Read the model definition and answer for the solid it produces. Units are mm, in the model's axes. Face numbers are marked on the shaded views. A direction names the side the tool comes from. Coordinates: 2 decimals unless noted, no trailing zeros. Order: outer loops, then holes, each group sorted by start corner. A loop starts at its lowest first (then second) coordinate and runs counter-clockwise, first axis right, second up. Notation, with made-up numbers: (-31, 42.25) - (-15, 42.25) arc R26 ccw to (-15, 63.25) - close; hole circle Ø3 at (-38, -29.75). An arc over 180 degrees is marked (long way). Use one line per item in the form item = value.
```python
from build123d import *

# Parameters (mm, degrees)
F0_W     = 155.6016728282
F0_H     = 72.8251989931
F1_DEPTH = 58.42
F2_W     = 155.6016728282
F2_H     = 9.92824696
F3_DEPTH = 25.4
F4_T     = 7.62
F5_R     = 5.08
F8_DEPTH = 25.4


# Not quite as in the source:
# - two fillets or chamfers of one size are made in one step
# - a shell that OpenCascade refuses in one call is made with other operations: the cavity is built on its own and cut out


with BuildPart() as f1:
    # F0 (on Front) → F1 (new body)
    with BuildSketch(Plane.XZ):
        with Locations((-1.8093250692, -6.1064558104)):
            Rectangle(F0_W, F0_H)
    extrude(amount=F1_DEPTH)

    # F2 (on face) → F3 (join)
    with BuildSketch(Plane.XY.offset(30.3061436862)):
        with Locations((-1.8093250692, -29.200729914)):
            Rectangle(F2_W, F2_H)
    extrude(amount=F3_DEPTH)

    # F4: shell of thickness 7.62, made by hand


with BuildPart() as f4_core1:
    # F4_t2: copy of F1
    add(f1.part)

    # the walls: a layer under each face that stays
    f4_faces = [f4_core1.faces().sort_by_distance(p)[0] for p in [
        (-1.8093250692, -12.118303217, 30.3061436862),
        (-1.8093250692, 0, -6.1064558104),
        (-79.6101614833, -29.21, 6.5935441896),
        (75.9915113449, -29.21, 6.5935441896),
        (-1.8093250692, -29.21, -42.5190553069),
        (-1.8093250692, -46.292426697, 30.3061436862),
        (-1.8093250692, -58.42, -6.1064558104),
        (-1.8093250692, -29.200729914, 55.7061436862),
    ]]
    thicken(f4_faces, amount=-F4_T, mode=Mode.SUBTRACT)


with BuildPart() as f1_1:
    add(f1.part)

    # what is left inside the walls is the cavity
    f4_cavity = [f4_core1.part.solids().sort_by_distance(p)[0] for p in [
        (-1.809325, -50.7238, -15.703989),
    ]]
    add(f4_cavity, mode=Mode.SUBTRACT)

    # F5
    f5_edges = [f1_1.edges().sort_by_distance(p)[0] for p in [
        (75.991511, -29.20073, 55.706144),
        (-79.610161, -29.20073, 55.706144),
    ]]
    fillet(f5_edges, radius=F5_R)

    # F7 (on face) → F8 (join)
    with BuildSketch(Plane(origin=(0, 0, 0), x_dir=(-1, 0, 0), z_dir=(0, 1, 0))):
        with BuildLine():
            Line((-33.5065312684, 8.8093429804), (-38.0396991968, 16.5818184614))
            ThreePointArc((-38.0396991968, 16.5818184614), (-46.9537485501, -29.5424136332), (0, -31.0426000506))
            ThreePointArc((0, -31.0426000506), (-11.7838373022, -4.7836219306), (-38.2480099797, -16.0991121083))
            ThreePointArc((-38.2480099797, -16.0991121083), (-40.6774615304, -20.5324220373), (-41.8258410886, -25.4556015134))
            ThreePointArc((-41.8258410886, -25.4556015134), (-44.7298971339, -6.6081053321), (-33.5065312684, 8.8093429804))
        make_face()
        with BuildLine():
            ThreePointArc((-31.2344189733, -35.0670516491), (-34.0695631474, -33.473512911), (-36.6739996827, -31.5256118532))
            ThreePointArc((-36.6739996827, -31.5256118532), (-36.1813498713, -25.629843598), (-33.3930179477, -20.4117987305))
            ThreePointArc((-33.3930179477, -20.4117987305), (-24.8135406655, -12.1786870208), (-12.9460245371, -12.9227433354))
            ThreePointArc((-12.9460245371, -12.9227433354), (-6.8355734632, -17.7428655691), (-5.7939905673, -25.4556015134))
            ThreePointArc((-5.7939905673, -25.4556015134), (-16.5679645446, -35.4128057466), (-31.2344189733, -35.0670516491))
        make_face(mode=Mode.SUBTRACT)
    extrude(amount=F8_DEPTH)


solid = f1_1.part
```
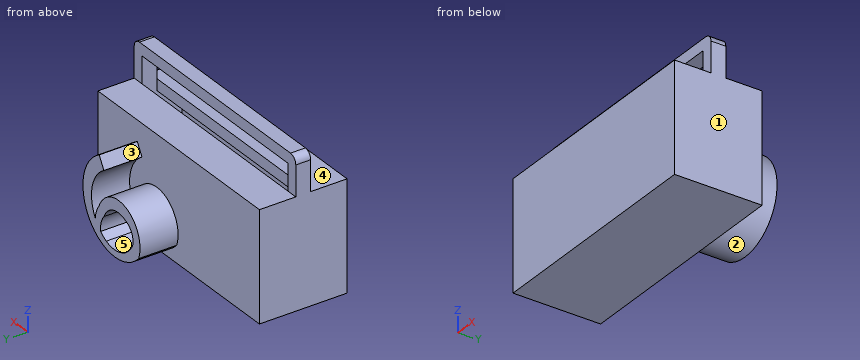
(1) Straight lines are drawn through the part: L1, parallel to Z at x = -71, y = -49.5; L2, parallel to X at y = -32.5, z = 17; L3, parallel to Y at x = 40, z = -13.5. For each, find the intervals that lie inside material, in ascending order.
Answer list:
L1 = -42.52 to -34.9, 22.69 to 30.31
L2 = -79.61 to -71.99, 68.37 to 75.99
L3 = -58.42 to -50.8, -7.62 to 0
(2) Section B-B, the plane x = -31.5 is taken. Write down the section's boundary in (y, z), then the cut area to 3 significant figures.
Answer list:
outline = (-58.42, -42.52) - (0, -42.52) - (0, 30.31) - (-24.24, 30.31) - (-24.24, 22.69) - (-7.62, 22.69) - (-7.62, -34.9) - (-50.8, -34.9) - (-50.8, 22.69) - (-34.16, 22.69) - (-34.16, 30.31) - (-58.42, 30.31) - close; (-34.16, 48.09) - (-24.24, 48.09) - (-24.24, 55.71) - (-34.16, 55.71) - close
area = 1,770 mm2
(3) Section D-D, the plane z = 1.5 is taken. Write down the section's boundary in (x, y).
Answer list:
outline = (-79.61, -58.42) - (75.99, -58.42) - (75.99, 0) - (51.37, 0) - (51.37, 25.4) - (41.14, 25.4) - (41.14, 0) - (-79.61, 0) - close; hole (-71.99, -50.8) - (68.37, -50.8) - (68.37, -7.62) - (-71.99, -7.62) - close
(4) Section C-C, the plane y = -42 is taken. Write down the section's boundary in (x, z).
Answer list:
outline = (-79.61, -42.52) - (75.99, -42.52) - (75.99, 30.31) - (-79.61, 30.31) - close; hole (-71.99, -34.9) - (68.37, -34.9) - (68.37, 22.69) - (-71.99, 22.69) - close
(5) The mould has two halves that part along X. Classify the marked faces 3, 4 and 5: +X half, -X half, draft (parallel to the pull), parting line (faces both ways), or undercut.
Answer list:
face_3 = -X half
face_4 = draft
face_5 = undercut
(6) Section A-A, the plane z = 43 is taken. Write down the section's boundary in (x, y), then the cut area to 3 significant figures.
Answer list:
outline = (-79.61, -34.16) - (-71.99, -34.16) - (-71.99, -24.24) - (-79.61, -24.24) - close; (68.37, -34.16) - (75.99, -34.16) - (75.99, -24.24) - (68.37, -24.24) - close
area = 151 mm2
(7) Given pin 1 Ø4 at (y, z) = (5.5, -6) entering from -X; pin 2 Ø7.5 at (x, y) = (18, -49.5) entering from +Z; pin 3 Ø20.5 at (x, z) = (10, 38.5) entering from +Y, each flat-ended and moving along its own axis, determine where each tip first touches the part or whether it passes through.
Answer list:
pin_1 = 6.27
pin_2 = 30.31
pin_3 = 0
(8) Which of the six approach directions +Z, -Z, +X, -X, +Y, -Y give full straight-line access (tool end or side, diameter ignored) to the marked faces 1 and 2?
Answer list:
face_1 = +Z, -Z, +X, +Y, -Y
face_2 = +Y
